```python
from build123d import *

# Parameters (mm, degrees)
SALIENTE_EXTRUIR1_DEPTH = 38.1
CROQUIS4_W              = 140.392352489
CROQUIS4_H              = 38.1
CORTAR_EXTRUIR2_DEPTH   = 6.31
CROQUIS5_W              = 38.1
CROQUIS5_H              = 6.31
SALIENTE_EXTRUIR2_DEPTH = 328.45


with BuildPart() as part:
    # Croquis1 → Saliente-Extruir1 (new body)
    with BuildSketch(Plane.XY):
        Polygon((0, 0), (202.937647511, 0), (202.937647511, 80), (349.64, 80), (349.64, 73.69), (209.247647511, 73.69), (209.247647511, -6.31), (0, -6.31), align=None)
    extrude(amount=SALIENTE_EXTRUIR1_DEPTH)

    # Croquis4 → Cortar-Extruir2 (cut)
    with BuildSketch(Plane.XZ.offset(-73.69)):
        with Locations((279.443823756, 19.05)):
            Rectangle(CROQUIS4_W, CROQUIS4_H)
    extrude(amount=-CORTAR_EXTRUIR2_DEPTH, mode=Mode.SUBTRACT)

    # Croquis5 → Saliente-Extruir2 (add)
    with BuildSketch(Plane.ZY):
        with Locations((19.05, -3.155)):
            Rectangle(CROQUIS5_W, CROQUIS5_H)
    extrude(amount=SALIENTE_EXTRUIR2_DEPTH)


solid = part.part
```
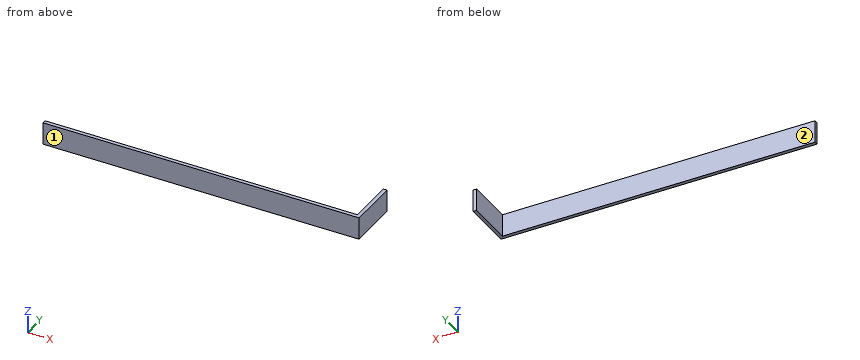
Work out the finished part from the listing and answer in its coordinate system (mm). Face numbers are marked on the shaded views. A direction names the side the tool comes from. Round coordinates to 2 decimals unless told otherwise and drop trailing zeros. Loops run counter-clockwise (first coordinate to the right, second up) from the corner with the lowest first, then second, coordinate; pieces in that order, holes last. Notation, with made-up numbers: (78, 55) -> (129, 55) arc R24 cw to (129, 86) -> close; hole circle Ø1 at (-24, 87.5). An arc over 180 degrees is marked (long way). Write each question's results on one line, items separated by ' | '. Start each with the question number.
1. Section B-B (y = 59) is taken. Determine the outline of the cut face in (x, z).
2. Section C-C (x = 54.5) is taken. Determine the outline of the cut face in (y, z).
3. Find the intervals of material crossed by probe 1 along Y at (x, z) = (128, 12.5); probe 2 along X at (y, z) = (55, 13.5), in increasing order. Write a range as from..to.
4. Given pin 1 Ø19 at (y, z) = (36.5, 22.5) entering from -X; pin 2 Ø3 at (x, z) = (132, 27.5) entering from +Y, each flat-ended and moving along its own axis, determine where each tip first touches the part or whether it passes through.
5. A tool of negligible diameter and unlimited length cuts with its end or side. For the marked faces 1 and 2, from which of +Z, -Z, +X, -X, +Y, -Y can it reach the whole face along a straight path? Write none if from no direction.
6. Section A-A (z = 11) is taken. Determine the outline of the cut face in (x, y).
Evaluation:
1) outline: (202.94, 0) -> (209.25, 0) -> (209.25, 38.1) -> (202.94, 38.1) -> close
2) outline: (-6.31, 0) -> (0, 0) -> (0, 38.1) -> (-6.31, 38.1) -> close
3) probe 1: y = -6.31..0 | probe 2: x = 202.94..209.25
4) pin 1: stops at x = 202.94 | pin 2: stops at y = 0
5) face 1: +Z, -Z, +X, -X, -Y | face 2: +Z, -Z, -X, +Y
6) outline: (-328.45, -6.31) -> (209.25, -6.31) -> (209.25, 80) -> (202.94, 80) -> (202.94, 0) -> (-328.45, 0) -> close
